Read the model definition and answer for the solid it produces. Units are mm, in the model's axes. Coordinates: 2 decimals unless noted, no trailing zeros. Loops run counter-clockwise (first coordinate to the right, second up) from the corner with the lowest first, then second, coordinate; pieces in that order, holes last. Notation, with made-up numbers: (64.5, 62) - (81.5, 62) arc R9 cw to (81.5, 73) - close; hole circle Ø9 at (-9, 36.25). An arc over 180 degrees is marked (long way). Use one line per item in the form item = value. Start each with the question number.
1) A cutting plane is placed at A-A (z = 1). Give the vertices of the cut face in (x, y) (3 decimals), and give its area (3 significant figures).
2) Consider line 1 (Y direction, x = 957, z = 4.75) (3 decimals); line 2 (Y direction, x = 685, z = -1.25) (3 decimals); line 3 (Z direction, x = 878, y = -2.25) (3 decimals). Determine where each line is inside the solid, lowest interval first.
3) A cutting plane is placed at C-C (y = 0.25). Give the vertices of the cut face in (x, z) (3 decimals), and give its area (3 significant figures).
4) This flat-tipped pin is pushed along its axis until it touches: P1, Ø3, axis at x = 917, y = 1.5, coming from the +Z side (3 decimals). Where does it stop, or does it pass through?
from build123d import *

# Parameters (mm, degrees)
F1_DEPTH = 1828.8


with BuildPart() as f1:
    # F0 (on Right) → F1 (new body)
    with BuildSketch(Plane.YZ):
        Polygon((-9.525, 6.35), (-9.525, -6.35), (9.525, -6.35), (9.525, 6.35), (3.175, 6.35), (3.175, 3.175), (6.35, 3.175), (6.35, -1.5875), (3.175, -1.5875), (3.175, -3.175), (-3.175, -3.175), (-3.175, -1.5875), (-6.35, -1.5875), (-6.35, 3.175), (-3.175, 3.175), (-3.175, 6.35), align=None)
    extrude(amount=F1_DEPTH)


solid = f1.part
Found:
q1.outline = (0, -9.525) - (1828.8, -9.525) - (1828.8, -6.35) - (0, -6.35) - close; (0, 6.35) - (1828.8, 6.35) - (1828.8, 9.525) - (0, 9.525) - close
q1.area = 11,600 mm^2
q2.line_1 = -9.525 to -3.175, 3.175 to 9.525
q2.line_2 = -9.525 to -6.35, 6.35 to 9.525
q2.line_3 = -6.35 to -3.175
q3.outline = (0, -6.35) - (1828.8, -6.35) - (1828.8, -3.175) - (0, -3.175) - close
q3.area = 5,810 mm^2
q4.P1 = -3.175
